Drawing for the job (mm, zero at the part's lowest x, y, z). Round coordinates to 2 decimals unless told otherwise and drop trailing zeros. Write each loop counter-clockwise with the first axis right and the second up, starting at its lowest first coordinate (ties: lowest second). Pieces come first, ordered by that corner, then holes. Notation, with made-up numbers: (83.5, -25) - (87.5, -25) arc R35 ccw to (87.5, 11) - close; hole circle Ø9 at (-26, 51). An arc over 180 degrees is marked (long way). Answer in a Markdown table with one row per item.
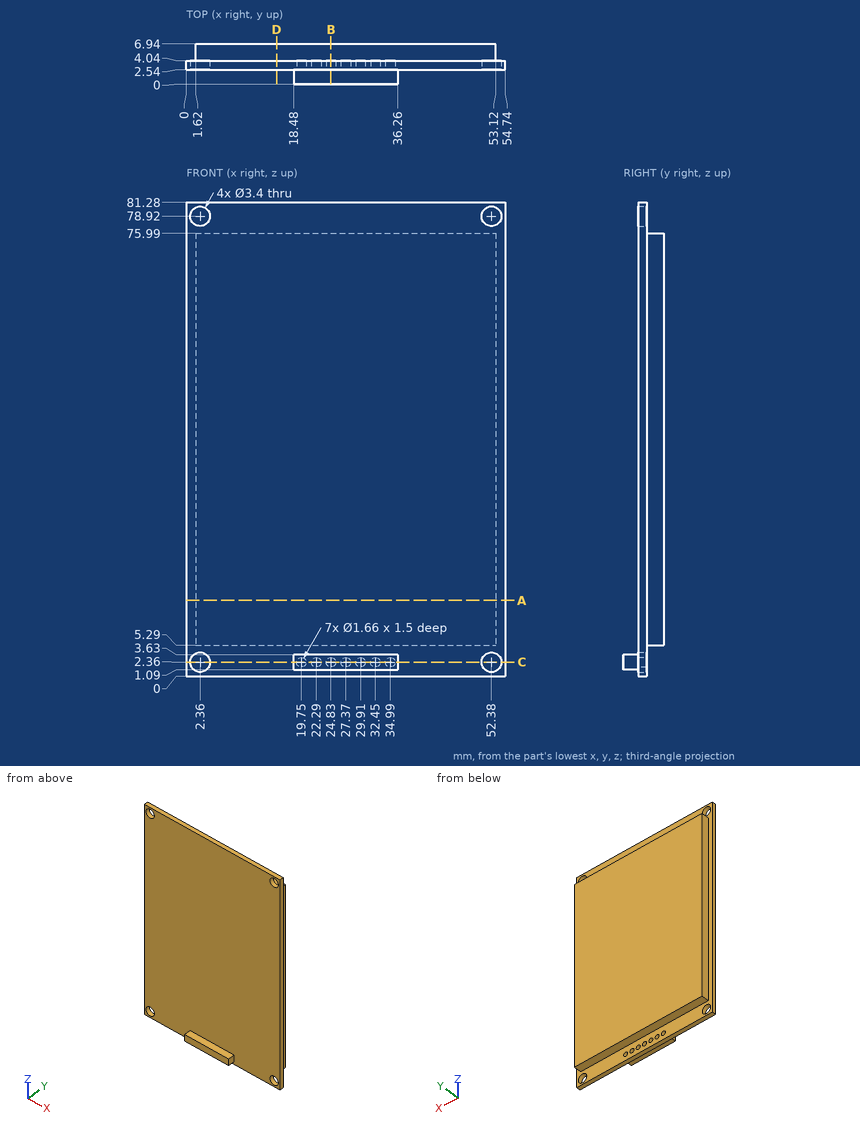
Q1. Drill centre lines: line 1 (X direction, y = 3.2, z = 78.92); line 2 (Y direction, x = 13.5, z = 19.5); line 3 (X direction, y = 4.25, z = 12). Where is each one in solid material? Low to high.
Computed:
| item | result |
|---|---|
| line 1 | x = 0 to 0.66, 4.06 to 50.68, 54.08 to 54.74 |
| line 2 | y = 2.54 to 6.94 |
| line 3 | x = 1.62 to 53.12 |
Q2. Saw through at C-C on z = 2.36. Count the separate pieces of the cut face and the enclosed holes in it, then the cut area to 3 significant figures.
Computed:
| item | result |
|---|---|
| separate pieces | 3 |
| enclosed holes | 0 |
| area | 99.6 mm2 |
Q3. Saw through at A-A on z = 13. List the corners of the cut face in (x, y), then the cut area to 3 significant figures.
Computed:
| item | result |
|---|---|
| outline | (0, 2.54) - (54.74, 2.54) - (54.74, 4.04) - (53.12, 4.04) - (53.12, 6.94) - (1.62, 6.94) - (1.62, 4.04) - (0, 4.04) - close |
| area | 231 mm2 |
Q4. Saw through at D-D on x = 15.5. List the corners of the cut face in (y, z), then the cut area to 3 significant figures.
Computed:
| item | result |
|---|---|
| outline | (2.54, 0) - (4.04, 0) - (4.04, 5.29) - (6.94, 5.29) - (6.94, 75.99) - (4.04, 75.99) - (4.04, 81.28) - (2.54, 81.28) - close |
| area | 327 mm2 |
Q5. Saw through at B-B on x = 24.83. List the corners of the cut face in (y, z), then the cut area to 3 significant figures.
Computed:
| item | result |
|---|---|
| outline | (0, 1.09) - (2.54, 1.09) - (2.54, 0) - (4.04, 0) - (4.04, 1.53) - (2.54, 1.53) - (2.54, 3.19) - (4.04, 3.19) - (4.04, 5.29) - (6.94, 5.29) - (6.94, 75.99) - (4.04, 75.99) - (4.04, 81.28) - (2.54, 81.28) - (2.54, 3.63) - (0, 3.63) - close |
| area | 331 mm2 |
Q6. Flat gauge pins, fed straight in: pin 1 (1 mm diameter, centred on x = 30, z = 27.5, fed in from -Y); pin 2 (0.5 mm diameter, centred on x = 22.5, z = 2, fed in from +Y); pin 3 (3 mm diameter, centred on x = 2.36, z = 2.36, fed in from -Y); pin 4 (0.9 mm diameter, centred on y = 6, z = 50.5, fed in from -X). Where does each tip first touch, or does it go through?
Computed:
| item | result |
|---|---|
| pin 1 | stops at y = 2.54 |
| pin 2 | stops at y = 2.54 |
| pin 3 | passes through |
| pin 4 | stops at x = 1.62 |
